Build history of the part. All positions in model axes, mm. Face numbers are marked on the shaded views. A direction names the side the tool comes from. Coordinates: 2 decimals unless noted, no trailing zeros. Write each loop counter-clockwise with the first axis right and the second up, starting at its lowest first coordinate (ties: lowest second). Pieces come first, ordered by that corner, then holes.
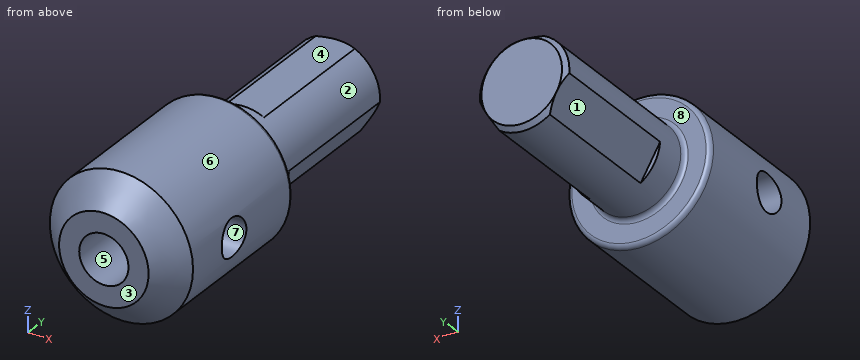
```python
from build123d import *

# Parameters (mm, degrees)
F0_R            = 8
F1_DEPTH        = 20
F2_R            = 5
F3_DEPTH        = 20
F5_DEPTH        = 16
F5_COPIES_COUNT = 3
F6_SIZE         = 0.49999
F7_R            = 0.5
F9_D            = 5.5
F9_DEPTH        = 14
F9_TIP          = 1.6523667023
F10_R           = 2.1
F11_DEPTH       = 8.25
F12_SIZE        = 3


# Not quite as in the source:
# - a fillet or chamfer is up to 0.001 mm smaller than in the source, because OpenCascade refuses the exact size
# - a pattern or mirror of a feature is missing from the dataset's text; its kind, count and spacing are read off the source's solid


with BuildPart() as f1:
    # F0 (on Front) → F1 (new body)
    with BuildSketch(Plane.XZ):
        Circle(F0_R)
    extrude(amount=-F1_DEPTH)

    # F2 (on face) → F3 (join)
    with BuildSketch(Plane(origin=(0, 20, 0), x_dir=(-1, 0, 0), z_dir=(0, 1, 0))):
        Circle(F2_R)
    extrude(amount=F3_DEPTH)

    # F4 (on face) → F5 (cut)
    with BuildSketch(Plane(origin=(0, 40, 0), x_dir=(-1, 0, 0), z_dir=(0, 1, 0))):
        with BuildLine():
            ThreePointArc((2.1794494718, 4.5), (0, 5), (-2.1794494718, 4.5))
            Line((-2.1794494718, 4.5), (2.1794494718, 4.5))
        make_face()
    f5 = extrude(amount=-F5_DEPTH, mode=Mode.SUBTRACT)

    # F5_copies: F5 ×3 about axis
    f5_copies_axis = Axis((0, 0, 0), (0, 1, 0))
    for i in range(1, F5_COPIES_COUNT):
        add(f5.rotate(f5_copies_axis, i * 360 / F5_COPIES_COUNT), mode=Mode.SUBTRACT)

    # F6 (size 0.5 in the source; OpenCascade refuses exactly that, so slightly less here)
    f6_edges = [f1.edges().sort_by_distance(p)[0] for p in [
        (4.330127, 40, 2.5),
        (-4.996709, 40, -0.18139),
        (0, 40, -5),
        (-4.236582, 40, 2.655443),
    ]]
    chamfer(f6_edges, length=F6_SIZE)

    # F7
    f7_edges = [f1.edges().sort_by_distance(p)[0] for p in [
        (-8, 20, 0),
        (5, 20, 0),
    ]]
    fillet(f7_edges, radius=F7_R)

    # F9
    with Locations(Plane.XZ):
        with Locations((0, 0)):
            Hole(F9_D / 2, depth=F9_DEPTH)
            with Locations((0, 0, -(F9_DEPTH + F9_TIP / 2))):  # 118° drill point
                Cone(0, F9_D / 2, F9_TIP, mode=Mode.SUBTRACT)

    # F10 (on Right) → F11 (cut, symmetric)
    with BuildSketch(Plane.YZ):
        with Locations((10, 0)):
            Circle(F10_R)
    extrude(amount=F11_DEPTH, both=True, mode=Mode.SUBTRACT)

    # F12
    f12_edges = [f1.edges().sort_by_distance(p)[0] for p in [
        (-8, 0, 0),
    ]]
    chamfer(f12_edges, length=F12_SIZE)


solid = f1.part
```
1. 3-axis set-ups, long thin cutter, end or side, ignore diameter. For the marked faces 1, 2, 3, 4 and 5: which of +Z, -Z, +X, -X, +Y, -Y reach the whole face in a straight line?
Computed values:
face 1: -Z, -X, +Y
face 2: +Y
face 3: +Z, -Z, +X, -X, -Y
face 4: +Z, +X, -X, +Y
face 5: -Y
2. Saw through at B-B on y = 32. List the corners of the cut face in (x, z).
Computed values:
outline: (-4.99, -0.36) - (-2.81, -4.14) arc R5 ccw to (2.81, -4.14) - (4.99, -0.36) arc R5 ccw to (2.18, 4.5) - (-2.18, 4.5) arc R5 ccw to start
3. Mould opens along Z. For the marked faces 6, 7 and 8 say: +Z half, -Z half, draft (parallel to the pull), parting line (faces both ways), or undercut.
Computed values:
face 6: parting line
face 7: undercut
face 8: draft
4. Probe line 1 along Z through (x, y) = (0, 5.5); line 2 along Y through (x, z) = (4.5, 0); line 3 along Y through (x, z) = (0, 0). List the from-to ranges inside material, lowest first.
Computed values:
line 1: z = -8 to -2.75, 2.75 to 8
line 2: y = 0 to 7.9, 12.1 to 40
line 3: y = 15.65 to 40
5. Flat gauge pins, fed straight in: pin 1 (1 mm diameter, centred on x = -2.5, y = 18, fed in from +Z); pin 2 (2 mm diameter, centred on x = -0.5, y = 34, fed in from +Z); pin 3 (1.5 mm diameter, centred on y = 25, z = 2.5, fed in from -X); pin 4 (4 mm diameter, centred on y = 10, z = 0, fed in from -X). Where does each tip first touch, or does it go through?
Computed values:
pin 1: stops at z = 7.75
pin 2: stops at z = 4.5
pin 3: stops at x = -4.68
pin 4: passes through
6. Saw through at C-C on y = 22. List the corners of the cut face in (x, z).
Computed values:
outline: circle Ø10 at (0, 0)
7. Saw through at A-A on y = 10. List the corners of the cut face in (x, z), plus the area to 3 significant figures.
Computed values:
outline: (-7.72, -2.1) arc R8 ccw to (7.72, -2.1) - (1.78, -2.1) arc R2.75 cw to (-1.78, -2.1) - close; (-7.72, 2.1) - (-1.78, 2.1) arc R2.75 cw to (1.78, 2.1) - (7.72, 2.1) arc R8 ccw to start
area: 131 mm2
